Here's how the part is built. I have some questions about the finished solid (model axes, mm). A direction names the side the tool comes from. Give positions to 0.01 mm unless a question says otherwise; leave off trailing zeros. Loops run counter-clockwise (first coordinate to the right, second up) from the corner with the lowest first, then second, coordinate; pieces in that order, holes last. Notation, with made-up numbers: (73.25, -13) - (107.25, -13) arc R22 ccw to (107.25, 11) - close; hole circle Ø9 at (52, 44.25). An arc over 180 degrees is marked (long way). One line per item, written item: value. Start each with the question number.
```python
from build123d import *

# Parameters (mm, degrees)
F0_W     = 1270
F0_H     = 762
F1_DEPTH = 19.05
F0_H_2   = 19.05
F2_DEPTH = 38.1
F3_R     = 6.35


with BuildPart() as f1:
    # F0 (on Top) → F1 (new body)
    with BuildSketch(Plane.XY):
        with Locations((-54.064326, 84.644601)):
            Rectangle(F0_W, F0_H)
    extrude(amount=F1_DEPTH)

    # F0 (on Top) → F2 (join)
    with BuildSketch(Plane.XY):
        Polygon((-689.064326, -296.355399), (-689.064326, 465.644601), (-708.114326, 465.644601), (-708.114326, -315.405399), (-689.064326, -315.405399), align=None)
        with Locations((-54.064326, -305.880399)):
            Rectangle(F0_W, F0_H_2)
        Polygon((599.985674, 465.644601), (580.935674, 465.644601), (580.935674, -296.355399), (580.935674, -315.405399), (599.985674, -315.405399), align=None)
    extrude(amount=F2_DEPTH)

    # F3
    f3_edges = [f1.edges().sort_by_distance(p)[0] for p in [
        (599.985674, 75.119601, 0),
        (-54.064326, -315.405399, 0),
        (-708.114326, 75.119601, 0),
        (-708.114326, 75.119601, 38.1),
        (-708.114326, -315.405399, 19.05),
        (-54.064326, -315.405399, 38.1),
        (599.985674, 75.119601, 38.1),
        (599.985674, -315.405399, 19.05),
    ]]
    fillet(f3_edges, radius=F3_R)


solid = f1.part
```
(1) For faces 1 (the face through (-63, 90, 19.05)), 2 (the face through (599.986, 73, 19)), which set-ups out of +Z, -Z, +X, -X, +Y, -Y let a thin tool reach every point of the face, with its end or its side?
(2) Please list where these lines run through material, in increasing order: probe 1 along Z at (x, y) = (-503.5, 210); probe 2 along Y at (x, z) = (-381, 20); probe 3 along X at (y, z) = (-263, 24.5). Write a range as from..to.
(3) Will these pins go through, and if not, where does the flat tip stop? pin 1 (10 mm diameter, centred on x = 71, y = 61.5, fed in from +Z); pin 2 (9.5 mm diameter, centred on x = 24, z = 33, fed in from +Y).
(4) If we section it at B-B on x = -244: List the corners of the cut face in (y, z) for me.
(5) If we section it at A-A on y = -74.5: List the corners of the cut face in (x, z) for me.
Found:
1. face 1: +Z, +Y
1. face 2: +Z, -Z, +X, +Y, -Y
2. probe 1: 0..19.05
2. probe 2: -315.41..-296.36
2. probe 3: -708.11..-689.06, 580.94..599.99
3. pin 1: z = 19.05
3. pin 2: y = -296.36
4. outline: (-315.41, 6.35) arc R6.35 ccw to (-309.06, 0) - (465.64, 0) - (465.64, 19.05) - (-296.36, 19.05) - (-296.36, 38.1) - (-309.06, 38.1) arc R6.35 ccw to (-315.41, 31.75) - close
5. outline: (-708.11, 6.35) arc R6.35 ccw to (-701.76, 0) - (593.64, 0) arc R6.35 ccw to (599.99, 6.35) - (599.99, 31.75) arc R6.35 ccw to (593.64, 38.1) - (580.94, 38.1) - (580.94, 19.05) - (-689.06, 19.05) - (-689.06, 38.1) - (-701.76, 38.1) arc R6.35 ccw to (-708.11, 31.75) - close
